```python
from build123d import *

# Parameters (mm, degrees)
SKICA1_W                 = 170
SKICA1_H                 = 170
P_IDAT_VYSUNUT_M1_DEPTH  = 1.57
SKICA2_R                 = 1.98
ODEBRAT_VYSUNUT_M1_DEPTH = 121.218404997
SKICA5_W                 = 74.714921367
SKICA5_H                 = 49.436852068
SKICA5_W_2               = 13.058822206
SKICA5_H_2               = 20.074329326
SKICA5_W_3               = 30.123299763
SKICA5_H_3               = 20.63009193
SKICA5_W_4               = 15.040102655
SKICA5_H_4               = 19.44386018
SKICA5_W_5               = 37.10064142
SKICA5_H_5               = 9.432366463
SKICA5_W_6               = 23.63246263
SKICA5_W_7               = 4.604120699
SKICA5_H_6               = 15.347068998
SKICA5_W_8               = 3.0694138
SKICA5_H_7               = 10.485045568
P_IDAT_VYSUNUT_M3_DEPTH  = 10


with BuildPart() as part:
    # Skica1 → Přidat vysunutím1 (new body)
    with BuildSketch(Plane(origin=(0, 0, 0), x_dir=(1, 0, 0), z_dir=(0, 1, 0))):
        Rectangle(SKICA1_W, SKICA1_H)
    extrude(amount=P_IDAT_VYSUNUT_M1_DEPTH)

    # Skica2 → Odebrat vysunutím1 (cut, through all)
    with BuildSketch(Plane(origin=(0, 1.57, 0), x_dir=(1, 0, 0), z_dir=(0, 1, 0))):
        with Locations(Location((-78.65, 74.84, 0), (0, 0, 270))):
            Circle(SKICA2_R)
        with Locations(Location((-78.65, -80.1, 0), (0, 0, 270))):
            Circle(SKICA2_R)
        with Locations(Location((78.83, -80.1, 0), (0, 0, 270))):
            Circle(SKICA2_R)
        with Locations(Location((78.83, 51.98, 0), (0, 0, 270))):
            Circle(SKICA2_R)
    extrude(amount=-ODEBRAT_VYSUNUT_M1_DEPTH, mode=Mode.SUBTRACT)

    # Skica5 → Přidat vysunutím3 (add)
    with BuildSketch(Plane(origin=(0, 1.57, 0), x_dir=(1, 0, 0), z_dir=(0, 1, 0))):
        with Locations((0.444909378, 15.224526197)):
            Rectangle(SKICA5_W, SKICA5_H)
        with Locations((-21.296441518, 78.962835337)):
            Rectangle(SKICA5_W_2, SKICA5_H_2)
        with Locations((13.764534228, 78.684954035)):
            Rectangle(SKICA5_W_3, SKICA5_H_3)
        with Locations((51.258042544, 79.27806991)):
            Rectangle(SKICA5_W_4, SKICA5_H_4)
        with Locations((-28.628364805, -72.809161969)):
            Rectangle(SKICA5_W_5, SKICA5_H_5)
        with Locations((31.921759901, -72.809161969)):
            Rectangle(SKICA5_W_6, SKICA5_H_5)
        with Locations((-61.75978641, -28.925932014)):
            Rectangle(SKICA5_W_7, SKICA5_H_6)
        with Locations((-52.295760528, -28.925932014)):
            Rectangle(SKICA5_W_8, SKICA5_H_6)
        with Locations((-61.75978641, -48.481841274)):
            Rectangle(SKICA5_W_7, SKICA5_H_7)
        with Locations((-52.295760528, -48.481841274)):
            Rectangle(SKICA5_W_8, SKICA5_H_7)
    extrude(amount=P_IDAT_VYSUNUT_M3_DEPTH)


solid = part.part
```
Work out the finished part from the listing and answer in its coordinate system (mm). A direction names the side the tool comes from. Round coordinates to 2 decimals unless told otherwise and drop trailing zeros. Order: outer loops, then holes, each group sorted by start corner. A loop starts at its lowest first (then second) coordinate and runs counter-clockwise, first axis right, second up.
Q1. The mould has two halves that part along Z. Classify faces 5 (the flat face through (20.106, 6, 73)), 6 (the flat face through (14, 6, -89)), 7 (the cylindrical face through (-78.563, 0.796, -76.818)): pulls with the +Z half, pulls with the -Z half, needs draft (parallel to the pull), parting line crosses it, or undercut.
Solution:
face 5: needs draft
face 6: pulls with the -Z half
face 7: undercut
Q2. A cutting plane is placed at C-C, the plane z = -74.84. Determine the outline of the cut face in (x, y).
Solution:
outline: (-85, 0) - (-80.63, 0) - (-80.63, 1.57) - (-85, 1.57) - close; (-76.67, 0) - (85, 0) - (85, 1.57) - (58.78, 1.57) - (58.78, 11.57) - (43.74, 11.57) - (43.74, 1.57) - (28.83, 1.57) - (28.83, 11.57) - (-1.3, 11.57) - (-1.3, 1.57) - (-14.77, 1.57) - (-14.77, 11.57) - (-27.83, 11.57) - (-27.83, 1.57) - (-76.67, 1.57) - close
Q3. A tool of negligible diameter and unlimited length cuts with its end or side. For faces 1 (the flat face through (-36.913, 6, -15)), 2 (the flat face through (-50.761, 6, 29)), 3 (the flat face through (0, 6, 9.494)), 4 (the flat face through (-59.458, 6, 29)), from which of +Z, -Z, +X, -X, +Y, -Y can it reach the whole face along a straight path? Write none if from no direction.
Solution:
face 1: -Z, -X, +Y
face 2: +Z, -Z, +X, +Y
face 3: +X, -X, +Y
face 4: +Z, -Z, +Y
Q4. A cutting plane is placed at A-A, the plane z = 80.1. Determine the outline of the cut face in (x, y).
Solution:
outline: (-85, 0) - (-80.63, 0) - (-80.63, 1.57) - (-85, 1.57) - close; (-76.67, 0) - (76.85, 0) - (76.85, 1.57) - (-76.67, 1.57) - close; (80.81, 0) - (85, 0) - (85, 1.57) - (80.81, 1.57) - close
Q5. A cutting plane is placed at D-D, the plane x = 25.5. Determine the outline of the cut face in (y, z), then the cut area to 3 significant figures.
Solution:
outline: (0, -85) - (1.57, -85) - (1.57, -89) - (11.57, -89) - (11.57, -68.37) - (1.57, -68.37) - (1.57, -39.94) - (11.57, -39.94) - (11.57, 9.49) - (1.57, 9.49) - (1.57, 68.09) - (11.57, 68.09) - (11.57, 77.53) - (1.57, 77.53) - (1.57, 85) - (0, 85) - close
area: 1,060 mm2
Q6. A cutting plane is placed at B-B, the plane x = -78.65. Determine the outline of the cut face in (y, z).
Solution:
outline: (0, -85) - (1.57, -85) - (1.57, -76.82) - (0, -76.82) - close; (0, -72.86) - (1.57, -72.86) - (1.57, 78.12) - (0, 78.12) - close; (0, 82.08) - (1.57, 82.08) - (1.57, 85) - (0, 85) - close
Q7. Find the intervals of material crossed by line 1 along X through (y, z) = (0.6, 80.1); line 2 along X through (y, z) = (9.5, -73); line 3 along Z through (x, y) = (22, 8.75), in increasing order.
Solution:
line 1: x = -85 to -80.63, -76.67 to 76.85, 80.81 to 85
line 2: x = -27.83 to -14.77, -1.3 to 28.83, 43.74 to 58.78
line 3: z = -89 to -68.37, -39.94 to 9.49, 68.09 to 77.53
Q8. Given pin 1 Ø6 at (y, z) = (7.5, 37.5) entering from -X; pin 2 Ø5 at (y, z) = (6, 49) entering from +X; pin 3 Ø1.5 at (x, z) = (62.5, -69) entering from +Y; pin 4 Ø5 at (x, z) = (9, -20) entering from -Y, each flat-ended and moving along its own axis, determine where each tip first touches the part or whether it passes through.
Solution:
pin 1: stops at x = -64.06
pin 2: stops at x = -50.76
pin 3: stops at y = 1.57
pin 4: stops at y = 0
